Input: part model. Units: mm. Frame: model coordinates. A direction names the side the tool comes from. Coordinates: 2 decimals unless noted, no trailing zeros. Write each loop counter-clockwise with the first axis right and the second up, starting at its lowest first coordinate (ties: lowest second). Pieces come first, ordered by that corner, then holes. Notation, with made-up numbers: (48.5, -38.5) - (55.5, -38.5) arc R10 ccw to (55.5, -32.5) - close; hole circle Ø4 at (84, 52). An arc over 180 degrees is marked (long way). Use a Markdown table: item, result. Add a question column.
Q1. Material intervals for probe 1 along Y at (x, z) = (55, 63.5); probe 2 along X at (y, z) = (37.5, 12); probe 3 along Z at (x, y) = (17, 37), sorted ascending. Write a range as from..to.
Q2. Set-up query: faces 1 (the face through (7.62, 129.71, 57.35)), 2 (the face through (35.56, 67, 31)), 3 (the face through (14, 39, 35.56)). Return all of +Z, -Z, +X, -X, +Y, -Y with unobstructed straight access to the full face (end or side cutting, diameter ignored); none if empty.
Q3. Section query A-A (x = 38.1). Return the cut outline in (y, z), then the cut area to 3 significant figures.
Q4. Mould query, pull axis X, two halves, no side actions, for faces 4 (the face through (38, 55, 0)), 5 (the face through (38, 137.16, 57)). Classes: released by +X, released by -X, zero draft, split by the parting line, or undercut.
Q5. Pin query (flat end, axial travel): P1, Ø2.5, axis at x = 37.5, z = 29, coming from the -Y side; P2, Ø10.5, axis at x = 21, y = 25, coming from the +Z side; P3, Ø8.5, axis at x = 47, z = 59, coming from the -Y side. Return the tip coordinate at first contact, or that it passes through.
Q6. Section query C-C (z = 20.32). Return the cut outline in (x, y), then the cut area to 3 significant figures.
Q7. Section query B-B (y = 38.1). Return the cut outline in (x, z), then the cut area to 3 significant figures.
Q8. Section query D-D (z = 46.5). Return the cut outline in (x, y), then the cut area to 3 significant figures.
from build123d import *

# Parameters (mm, degrees)
F1_DEPTH = 76.2
F4_DEPTH = 10.16
F6_R     = 7.62
F7_DEPTH = 25.401
F2_R     = 10.16
F8_DEPTH = 76.201
F9_DEPTH = 27.94


with BuildPart() as f1:
    # F0 (on Right) → F1 (new body)
    with BuildSketch(Plane.YZ):
        Polygon((0, 35.56), (0, 0), (111.76, 0), (147.32, 35.56), (147.32, 71.12), (111.76, 71.12), (76.2, 35.56), align=None)
    extrude(amount=F1_DEPTH)

    # F3 (on face) → F4 (cut)
    with BuildSketch(Plane.XY.offset(35.56)):
        with BuildLine():
            Line((35.56, 76.2), (35.56, 58.260625))
            ThreePointArc((35.56, 58.260625), (17.78, 38.1), (35.56, 17.939375))
            Line((35.56, 17.939375), (35.56, 0))
            Line((35.56, 0), (40.64, 0))
            Line((40.64, 0), (40.64, 17.939375))
            ThreePointArc((40.64, 17.939375), (58.42, 38.1), (40.64, 58.260625))
            Line((40.64, 58.260625), (40.64, 76.2))
            Line((40.64, 76.2), (35.56, 76.2))
        make_face()
    extrude(amount=-F4_DEPTH, mode=Mode.SUBTRACT)

    # F6 (on face) → F7 (cut, through all)
    with BuildSketch(Plane.XY.offset(25.4)):
        with Locations((38.1, 38.1)):
            Circle(F6_R)
    extrude(amount=-F7_DEPTH, mode=Mode.SUBTRACT)

    # F2 (on face) → F8 (cut, through all)
    with BuildSketch(Plane.YZ.offset(76.2)):
        with Locations((93.98, 20.32)):
            Circle(F2_R)
    extrude(amount=-F8_DEPTH, mode=Mode.SUBTRACT)

    # F5 (on face) → F9 (cut)
    with BuildSketch(Plane.XY.offset(71.12)):
        with BuildLine():
            Line((60.96, 137.16), (15.24, 137.16))
            ThreePointArc((15.24, 137.16), (7.62, 129.54), (15.24, 121.92))
            Line((15.24, 121.92), (60.96, 121.92))
            ThreePointArc((60.96, 121.92), (68.58, 129.54), (60.96, 137.16))
        make_face()
    extrude(amount=-F9_DEPTH, mode=Mode.SUBTRACT)


solid = f1.part
Values follow:
| question | item | result |
|---|---|---|
| 1 | probe 1 | 104.14..121.92, 137.16..147.32 |
| 1 | probe 2 | 0..30.5, 45.7..76.2 |
| 1 | probe 3 | 0..35.56 |
| 2 | face 1 | +Z |
| 2 | face 2 | +Z, -Y |
| 2 | face 3 | +Z, +X, -X, -Y |
| 3 | outline | (0, 0) - (30.48, 0) - (30.48, 25.4) - (0, 25.4) - close; (45.72, 0) - (111.76, 0) - (147.32, 35.56) - (147.32, 71.12) - (137.16, 71.12) - (137.16, 43.18) - (121.92, 43.18) - (121.92, 71.12) - (111.76, 71.12) - (76.2, 35.56) - (76.2, 25.4) - (45.72, 25.4) - close; hole circle Ø20.32 at (93.98, 20.32) |
| 3 | area | 4,590 mm2 |
| 4 | face 4 | zero draft |
| 4 | face 5 | undercut |
| 5 | P1 | y = 76.2 |
| 5 | P2 | z = 35.56 |
| 5 | P3 | y = 95.39 |
| 6 | outline | (0, 0) - (76.2, 0) - (76.2, 83.82) - (0, 83.82) - close; (0, 104.14) - (76.2, 104.14) - (76.2, 132.08) - (0, 132.08) - close; hole circle Ø15.24 at (38.1, 38.1) |
| 6 | area | 8,330 mm2 |
| 7 | outline | (0, 0) - (30.48, 0) - (30.48, 25.4) - (17.78, 25.4) - (17.78, 35.56) - (0, 35.56) - close; (45.72, 0) - (76.2, 0) - (76.2, 35.56) - (58.42, 35.56) - (58.42, 25.4) - (45.72, 25.4) - close |
| 7 | area | 1,910 mm2 |
| 8 | outline | (0, 87.14) - (76.2, 87.14) - (76.2, 147.32) - (0, 147.32) - close; hole (15.24, 121.92) - (60.96, 121.92) arc R7.62 ccw to (60.96, 137.16) - (15.24, 137.16) arc R7.62 ccw to start |
| 8 | area | 3,710 mm2 |
